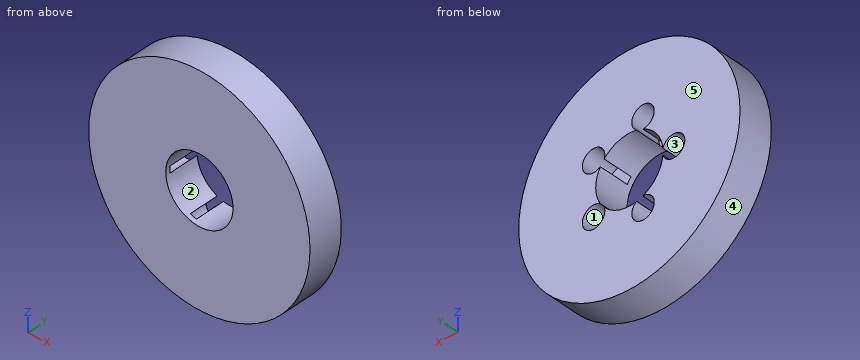
from build123d import *

# Parameters (mm, degrees)
SKETCH1_R           = 57.5
BOSS_EXTRUDE1_DEPTH = 18
SKETCH2_R           = 17.5
CUT_EXTRUDE1_DEPTH  = 84.285653026
SKETCH3_R           = 5.835493776
CUT_EXTRUDE2_DEPTH  = 15.493779
CIRPATTERN1_START   = 2.506221228
CIRPATTERN1_DEPTH   = 15.493778772


# Read off the part's stored shape, not the designer's step: CirPattern1
with BuildPart() as part:
    # Sketch1 → Boss-Extrude1 (new body)
    with BuildSketch(Plane(origin=(0, 0, 0), x_dir=(1, 0, 0), z_dir=(0, 1, 0))):
        with Locations(Location((0, 0, 0), (0, 0, 270))):
            Circle(SKETCH1_R)
    extrude(amount=BOSS_EXTRUDE1_DEPTH)

    # Sketch2 → Cut-Extrude1 (cut, through all)
    with BuildSketch(Plane(origin=(0, 0, 0), x_dir=(1, 0, 0), z_dir=(0, 1, 0))):
        with Locations(Location((0, 0, 0), (0, 0, 270))):
            Circle(SKETCH2_R)
    extrude(amount=CUT_EXTRUDE1_DEPTH, mode=Mode.SUBTRACT)

    # Sketch3 → Cut-Extrude2 (cut)
    with BuildSketch(Plane(origin=(0, 18, 0), x_dir=(1, 0, 0), z_dir=(0, 1, 0))):
        with Locations((-23.003411052, 0)):
            Circle(SKETCH3_R)
    extrude(amount=-CUT_EXTRUDE2_DEPTH, mode=Mode.SUBTRACT)

    # CirPattern1 outline → CirPattern1 (cut)
    with BuildSketch(Plane(origin=(0, 0, 0), x_dir=(1, 0, 0), z_dir=(0, 1, 0)).offset(CIRPATTERN1_START)):
        with BuildLine():
            ThreePointArc((-3.774714909, -17.088052181), (-5.407797402, -16.643489035), (-6.990296553, -16.04324637))
            ThreePointArc((-6.990296553, -16.04324637), (-8.911711691, -27.427428359), (-3.774714909, -17.088052181))
        make_face()
        with BuildLine():
            ThreePointArc((-3.774714909, 17.088052182), (-8.911711691, 27.427428359), (-6.990296553, 16.043246371))
            ThreePointArc((-6.990296553, 16.043246371), (-5.407797402, 16.643489035), (-3.774714909, 17.088052182))
        make_face()
        with BuildLine():
            ThreePointArc((15.085252322, -8.870465736), (14.157797401, -10.286241915), (13.097913573, -11.605802861))
            ThreePointArc((13.097913573, -11.605802861), (23.331164106, -16.951082949), (15.085252322, -8.870465736))
        make_face()
        with BuildLine():
            ThreePointArc((15.085252322, 8.870465736), (23.331164106, 16.951082949), (13.097913573, 11.605802861))
            ThreePointArc((13.097913573, 11.605802861), (14.157797401, 10.286241915), (15.085252322, 8.870465736))
        make_face()
    extrude(amount=CIRPATTERN1_DEPTH, mode=Mode.SUBTRACT)


solid = part.part
Input: part model. Units: mm. Frame: model coordinates. Face numbers are marked on the shaded views. A direction names the side the tool comes from. Give positions to 0.01 mm unless a question says otherwise; leave off trailing zeros. Order: outer loops, then holes, each group sorted by start corner. A loop starts at its lowest first (then second) coordinate and runs counter-clockwise, first axis right, second up. Notation, with made-up numbers: M 16,-14 L 56,-14 A25 cw 56,-1 Z; hole C -29.75,43.25 d6. An arc over 180 degrees is marked long. Answer as a JSON object with one key per item and string values.
1. Reachability of the marked faces 1 and 2 from +Z, -Z, +X, -X, +Y, -Y: full face, straight path, thin tool, end or side. Return the list, or none.
Result sheet:
{"face 1": "+Y", "face 2": "+Y, -Y"}
2. First-contact query: P1, Ø7, axis at x = 18.61, z = -13.52, coming from the +Y side; P2, Ø8, axis at x = 43.5, y = 2.5, coming from the -Z side; P3, Ø1, axis at x = -5, y = 2.5, coming from the +Z side. Flat tips, straight axial feed; report the tip coordinate or a pass-through.
Result sheet:
{"P1": "y = 2.51", "P2": "z = -41.79", "P3": "z = 57.32"}
3. Cut plane C-C, the plane x = -9. Output: boundary loops of the cut face in (y, z).
Result sheet:
{"outline": "M 0,-56.79 L 18,-56.79 L 18,-27.4 L 2.51,-27.4 L 2.51,-16.36 L 18,-16.36 L 18,-15.01 L 0,-15.01 Z; M 0,15.01 L 18,15.01 L 18,16.36 L 2.51,16.36 L 2.51,27.4 L 18,27.4 L 18,56.79 L 0,56.79 Z"}
4. Cut plane A-A, the plane z = 0. Output: boundary loops of the cut face in (x, y).
Result sheet:
{"outline": "M -57.5,0 L -17.5,0 L -17.5,2.51 L -28.84,2.51 L -28.84,18 L -57.5,18 Z; M 17.5,0 L 57.5,0 L 57.5,18 L 17.5,18 Z"}
5. Cut plane D-D, the plane x = -24. Output: boundary loops of the cut face in (y, z).
Result sheet:
{"outline": "M 0,-52.25 L 18,-52.25 L 18,-5.75 L 2.51,-5.75 L 2.51,5.75 L 18,5.75 L 18,52.25 L 0,52.25 Z"}
6. Pull-direction query (X, two-part tool) for the marked faces 3, 4 and 5; classes: +X half, -X half, draft (parallel to the pull), parting line (faces both ways), or undercut.
Result sheet:
{"face 3": "undercut", "face 4": "parting line", "face 5": "draft"}
7. Ray query, line 1 (Z direction, x = -2.5, y = 11.5); line 2 (Y direction, x = 13.5, z = 15.5); line 3 (Z direction, x = -5, y = 9.25). Return the intervals inside material, ascending. Write a range as [from, to].
Result sheet:
{"line 1": "[-57.45, -25.46], [-18.3, -17.32], [17.32, 18.3], [25.46, 57.45]", "line 2": "[0, 2.51]", "line 3": "[-57.28, -27.32], [27.32, 57.28]"}
8. Cut plane B-B, the plane y = 11. Output: boundary loops of the cut face in (x, z), and give its area (3 significant figures).
Result sheet:
{"outline": "C 0,0 d115; hole M -17.42,-1.69 A17.5 ccw -6.99,-16.04 A5.84 ccw long -3.77,-17.09 A17.5 ccw 13.1,-11.61 A5.84 ccw long 15.09,-8.87 A17.5 ccw 15.09,8.87 A5.84 ccw long 13.1,11.61 A17.5 ccw -3.77,17.09 A5.84 ccw long -6.99,16.04 A17.5 ccw -17.42,1.69 A5.84 ccw long Z", "area": "8,890 mm²"}
